For this review, use the dimensioned drawing (mm, ordinates from the lowest corner) and the shaded views. A direction names the side the tool comes from. Give positions to 0.01 mm unless a question says otherwise; leave off trailing zeros. Write each loop counter-clockwise with the first axis right and the second up, starting at its lowest first coordinate (ties: lowest second). Pieces come first, ordered by that corner, then holes. Notation, with made-up numbers: M 1,67.5 L 13,67.5 A17 cw 13,86.5 Z; hole C 50,23 d1. An arc over 180 degrees is marked long. Use a Markdown table: item, result. Add a question column.
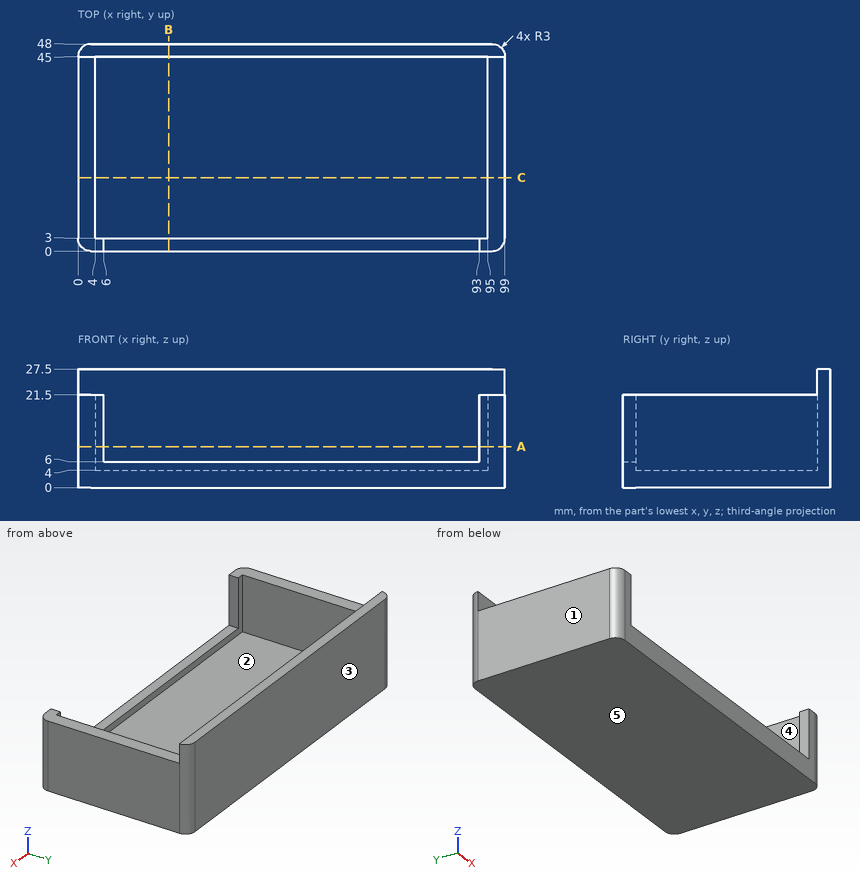
(1) For pin 1 (1.8 mm diameter, centred on x = 2.5, y = 25, fed in from +Z); pin 2 (0.9 mm diameter, centred on y = 1, z = 15, fed in from +X); pin 3 (4 mm diameter, centred on x = 41, z = 19, fed in from -Y), all flat-tipped, find the tip position at first contact; note any pin that passes through.
(2) Machinability: for the marked faces 4 and 5, which of the approach directions +Z, -Z, +X, -X, +Y, -Y give a long, thin tool a straight path to every point of the face, cutting with its end or side? Answer none if there is none.
(3) Add section C-C on y = 17. Give the boundary of the cut face in (x, z), then the cut area to 3 significant figures.
(4) Add section A-A on z = 9.5. Give the boundary of the cut face in (x, y), then the cut area to 3 significant figures.
(5) Wall thickness on L1, parallel to X at y = 18, z = 8.25; L2, parallel to Y at x = 23, z = 9.25; L3, parallel to Z at x = 23, y = 25: over which ranges is each line inside the solid? List them lowest first.
(6) Add section B-B on x = 21. Give the boundary of the cut face in (y, z), then the cut area to 4 significant figures.
(7) The part is to be moulded in two halves that separate along X. For the marked faces 1, 2 and 3, say which applies: released by +X, released by -X, zero draft, split by the parting line, or undercut.
From the geometry:
| question | item | result |
|---|---|---|
| 1 | pin 1 | stops at z = 21.5 |
| 1 | pin 2 | stops at x = 98.57 |
| 1 | pin 3 | stops at y = 45 |
| 2 | face 4 | +Z |
| 2 | face 5 | -Z, +X, -X, +Y, -Y |
| 3 | outline | M 0,0 L 99,0 L 99,21.5 L 95,21.5 L 95,4 L 4,4 L 4,21.5 L 0,21.5 Z |
| 3 | area | 536 mm^2 |
| 4 | outline | M 0,3 A3 ccw 3,0 L 6,0 L 6,3 L 4,3 L 4,45 L 95,45 L 95,3 L 93,3 L 93,0 L 96,0 A3 ccw 99,3 L 99,45 A3 ccw 96,48 L 3,48 A3 ccw 0,45 Z |
| 4 | area | 661 mm^2 |
| 5 | L1 | x = 0 to 4, 95 to 99 |
| 5 | L2 | y = 45 to 48 |
| 5 | L3 | z = 0 to 4 |
| 6 | outline | M 0,0 L 48,0 L 48,27.5 L 45,27.5 L 45,4 L 3,4 L 3,6 L 0,6 Z |
| 6 | area | 268.5 mm^2 |
| 7 | face 1 | released by -X |
| 7 | face 2 | undercut |
| 7 | face 3 | zero draft |
